Geometry check sheet. Reference: the model listing, model coordinates, mm. Face numbers are marked on the shaded views. A direction names the side the tool comes from. Round coordinates to 2 decimals unless told otherwise and drop trailing zeros. Order: outer loops, then holes, each group sorted by start corner. A loop starts at its lowest first (then second) coordinate and runs counter-clockwise, first axis right, second up. Notation, with made-up numbers: (72, -18) - (126, -18) arc R6 cw to (126, -9) - close; hole circle Ø9 at (53, -29.5). An arc over 180 degrees is marked (long way). Return JSON: item names as keys, results as strings. Group by question number.
Q1. Material ranges on line 1 along Y through (x, z) = (-91, 59); line 2 along Z through (x, y) = (-89.5, -15.5); line 3 along Z through (x, y) = (-101, -23.5), recorded low to high.
Q2. Sectioned sample at C-C, the plane y = -26.5. Give the number of separate pieces and of enclosed holes in the cut face, then the cut area to 3 significant figures.
Q3. Gauge pin test, flat ends, axial feed: pin 1 Ø1 at (y, z) = (-18.5, 20) entering from -X; pin 2 Ø3.5 at (x, z) = (-78, 78.5) entering from -Y; pin 3 Ø2 at (x, z) = (-71, 30) entering from +Y. Record the tip position at first contact, or that the pin passes through.
Q4. Tool access check on the marked faces 5, 6 and 7. Record the directions out of +Z, -Z, +X, -X, +Y, -Y that give a thin tool (end or side, any length) a straight path to the whole face; none if there is none.
Q5. Sectioned sample at B-B, the plane x = -49. Record the cut outline in (y, z).
Q6. Draft check along X on the marked faces 1, 2, 3 and 4. Enter one of: pulls with the +X half, pulls with the -X half, needs draft (parallel to the pull), parting line crosses it, or undercut.
Q7. Sectioned sample at A-A, the plane z = 69. Record the cut outline in (x, y), then the cut area to 3 significant figures.
```python
from build123d import *

# Parameters (mm, degrees)
SKETCH009_R             = 16.5
SKETCH009_R_2           = 2
PAD006_DEPTH            = 3
SKETCH010_R             = 1.5
PAD007_DEPTH            = 25
POLARPATTERN_COUNT      = 9
PAD008_DEPTH            = 25
SKETCH012_R             = 21.5
SKETCH012_R_2           = 18.7
SKETCH012_R_3           = 2.1
PAD009_DEPTH            = 2
PAD010_DEPTH            = 8.5
SKETCH014_R             = 2.8
PAD011_DEPTH            = 2.6
BODY004_PLACEMENT_ANGLE = 90


with BuildPart() as part:
    # Sketch009 → Pad006 (new body)
    with BuildSketch(Plane.YZ):
        Circle(SKETCH009_R)
        with Locations((0, 12)):
            Circle(SKETCH009_R_2, mode=Mode.SUBTRACT)
        with Locations((-6, 10.392305)):
            Circle(SKETCH009_R_2, mode=Mode.SUBTRACT)
        with Locations((6, 10.392305)):
            Circle(SKETCH009_R_2, mode=Mode.SUBTRACT)
        with Locations((12, 0)):
            Circle(SKETCH009_R_2, mode=Mode.SUBTRACT)
        with Locations((10.392305, -6)):
            Circle(SKETCH009_R_2, mode=Mode.SUBTRACT)
        with Locations((6, -10.392305)):
            Circle(SKETCH009_R_2, mode=Mode.SUBTRACT)
        with Locations((-6, -10.392305)):
            Circle(SKETCH009_R_2, mode=Mode.SUBTRACT)
        with Locations((-10.392305, -6)):
            Circle(SKETCH009_R_2, mode=Mode.SUBTRACT)
        with Locations((-12, 0)):
            Circle(SKETCH009_R_2, mode=Mode.SUBTRACT)
    extrude(amount=PAD006_DEPTH)

    # Sketch010 → Pad007 (join)
    with BuildSketch(Plane.YZ):
        with BuildLine():
            ThreePointArc((5.510568, -35.069697), (0, 35.5), (-5.510568, -35.069697))
            ThreePointArc((-2.988125, -37.766667), (-3.785221, -35.984091), (-5.510568, -35.069697))
            ThreePointArc((-2.988125, -37.766667), (0, -40.5), (2.988125, -37.766667))
            ThreePointArc((5.510568, -35.069697), (3.785221, -35.984091), (2.988125, -37.766667))
        make_face()
        with Locations((0, -37.5)):
            Circle(SKETCH010_R, mode=Mode.SUBTRACT)
    pad007 = extrude(amount=-PAD007_DEPTH)

    # PolarPattern: Pad007 ×9 about axis
    polarpattern_axis = Axis((0, 0, 0), (1, 0, 0))
    for i in range(1, POLARPATTERN_COUNT):
        add(pad007.rotate(polarpattern_axis, i * 360 / POLARPATTERN_COUNT))

    # Sketch011 → Pad008 (join)
    with BuildSketch(Plane.YZ):
        with BuildLine():
            ThreePointArc((-6.626667, 34.876027), (-5.459437, 35.565466), (-5, 36.840874))
            Line((-5, 37.840874), (-5, 36.840874))
            ThreePointArc((-3, 39.840874), (-4.414214, 39.255088), (-5, 37.840874))
            Line((-3, 39.840874), (3, 39.840874))
            ThreePointArc((5, 37.840874), (4.414214, 39.255088), (3, 39.840874))
            Line((5, 37.840874), (5, 36.840874))
            ThreePointArc((5, 36.840874), (5.459437, 35.565466), (6.626667, 34.876027))
            ThreePointArc((6.626667, 34.876027), (0, 35.5), (-6.626667, 34.876027))
        make_face()
    extrude(amount=-PAD008_DEPTH)

    # Sketch012 → Pad009 (join)
    with BuildSketch(Plane.YZ):
        Circle(SKETCH012_R)
        Circle(SKETCH012_R_2, mode=Mode.SUBTRACT)
        with Locations((0, 29)):
            Circle(SKETCH012_R_3)
    extrude(amount=PAD009_DEPTH)

    # Sketch013 → Pad010 (join)
    with BuildSketch(Plane.YZ.offset(-25)):
        with BuildLine():
            ThreePointArc((-7, 30.712375), (0, -31.5), (7, 30.712375))
            Line((7, 36.5), (7, 30.712375))
            Line((-7, 36.5), (7, 36.5))
            Line((-7, 30.712375), (-7, 36.5))
        make_face()
    extrude(amount=-PAD010_DEPTH)

    # Sketch014 → Pad011 (join)
    with BuildSketch(Plane.YZ.offset(-25)):
        with Locations((0, -37.5)):
            Circle(SKETCH014_R)
        with Locations((32.475953, 18.75)):
            Circle(SKETCH014_R)
        with Locations((-32.475953, 18.75)):
            Circle(SKETCH014_R)
    extrude(amount=-PAD011_DEPTH)


with BuildPart() as part_1:
    # Body004 placement: moved
    add(part.part.moved(Location((-77.6, -10, 40))).rotate(Axis((-77.6, -10, 40), (0, 0, 1)), BODY004_PLACEMENT_ANGLE))


solid = part_1.part
```
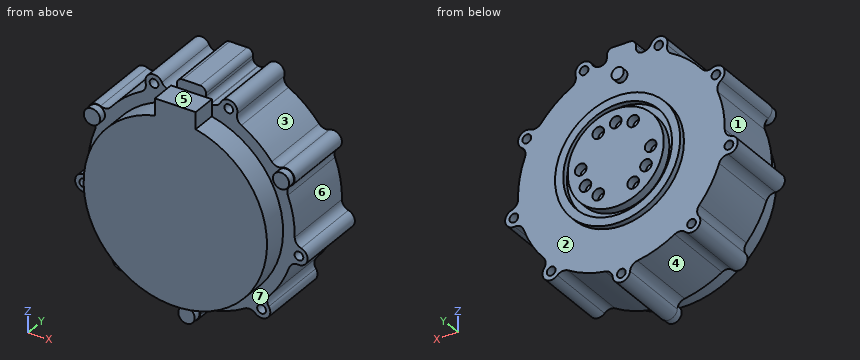
Reply:
{
 "1": {"line 1": "-43.5 to -10", "line 2": "6.55 to 74.06, 76.42 to 78.09", "line 3": "8.36 to 9.95, 12.6 to 66.7"},
 "2": {"separate pieces": "1", "enclosed holes": "9", "area": "4,200 mm^2"},
 "3": {"pin 1": "x = -107.26", "pin 2": "y = -35", "pin 3": "y = -10"},
 "4": {"face 5": "+Z, +X, -X, -Y", "face 6": "+X, +Y, -Y", "face 7": "-Y"},
 "5": {"outline": "(-43.5, 26.8) - (-35, 26.8) - (-35, 18.97) - (-10, 18.97) - (-10, 61.51) - (-35, 61.51) - (-35, 53.2) - (-43.5, 53.2) - close"},
 "6": {"face 1": "pulls with the -X half", "face 2": "needs draft", "face 3": "pulls with the +X half", "face 4": "undercut"},
 "7": {"outline": "(-98.08, -35) - (-89.9, -35) - (-89.9, -43.5) - (-65.3, -43.5) - (-65.3, -35) - (-57.12, -35) - (-57.12, -10) - (-75.5, -10) - (-75.5, -8) - (-79.7, -8) - (-79.7, -10) - (-98.08, -10) - close", "area": "1,240 mm^2"}
}
